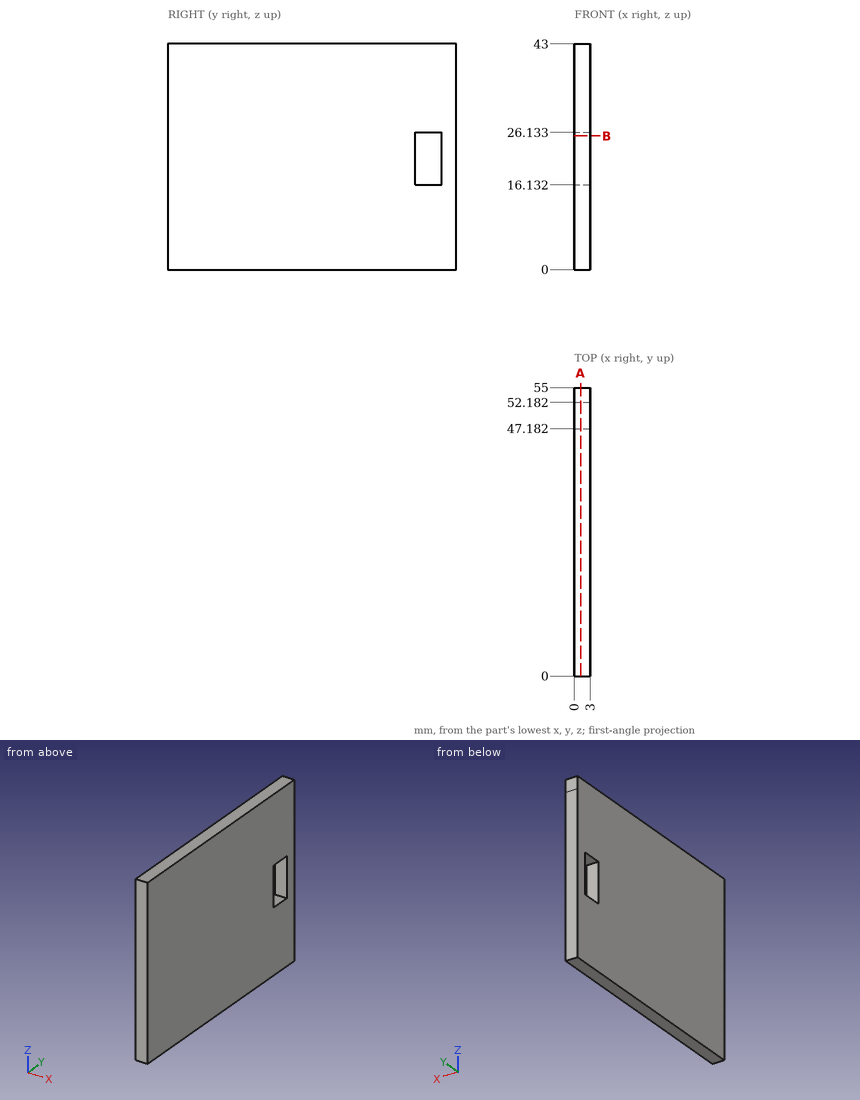
Here's the drawing with two shaded views (mm, measured from the low corner). I have some questions. Coordinates: 2 decimals unless noted, no trailing zeros. Order: outer loops, then holes, each group sorted by start corner. A loop starts at its lowest first (then second) coordinate and runs counter-clockwise, first axis right, second up.
Item 1: I need wall thicknesses on probe 1 along Y at (x, z) = (2.8, 23); probe 2 along Z at (x, y) = (1.5, 49). Which ranges of each line are inside material? Lowest first, please.
Response values:
probe 1: y = 0 to 47.18, 52.18 to 55
probe 2: z = 0 to 16.13, 26.13 to 43
Item 2: If we section it at A-A, the plane x = 1.2: List the corners of the cut face in (y, z) for me, then the cut area to 4 significant figures.
Response values:
outline: (0, 0) - (55, 0) - (55, 40) - (55, 43) - (0, 43) - close; hole (47.18, 16.13) - (52.18, 16.13) - (52.18, 26.13) - (47.18, 26.13) - close
area: 2,315 mm2
Item 3: If we section it at B-B, the plane z = 25.5: List the corners of the cut face in (x, y) for me.
Response values:
outline: (0, 0) - (3, 0) - (3, 47.18) - (0, 47.18) - close; (0, 52.18) - (3, 52.18) - (3, 55) - (0, 55) - close
